Source: CAD feature listing. Evaluate the final solid. Frame: model axes, mm. Face numbers are marked on the shaded views. A direction names the side the tool comes from. Give positions to 0.01 mm unless a question says otherwise; leave off trailing zeros. Loops run counter-clockwise (first coordinate to the right, second up) from the corner with the lowest first, then second, coordinate; pieces in that order, holes last. Notation, with made-up numbers: (56.25, -37.5) - (85.25, -37.5) arc R31 ccw to (85.25, -11.5) - close; hole circle Ø8 at (31.5, -4). An arc over 180 degrees is marked (long way). Put each result on its own line as item: value.
```python
from build123d import *

# Parameters (mm, degrees)
ESBO_O3_W                  = 13.686755529
ESBO_O3_H                  = 42.535935493
ESBO_O4_W                  = 38.680905152
ESBO_O4_H                  = 38.535935493
CORTE_EXTRUS_O1_DEPTH      = 1635.545265364
CORTE_EXTRUS_O1_DEPTH_BACK = 1635.545265364
ESBO_O6_R                  = 34.061990031
ESBO_O7_W                  = 13.69
ESBO_O7_H                  = 42.54
ESBO_O8_W                  = 38.68
ESBO_O8_H                  = 38.54


with BuildPart() as part:
    # Esboço1 → Revolução6 (revolve)
    with BuildSketch(Plane.XY, mode=Mode.PRIVATE) as revolu_o6_sk:
        Polygon((0, 1633), (-35.838224288, 1633), (-35.838224288, 1534.993249603), (-50.245519822, 1534.993249603), (-50.245519822, 1398.116209781), (-35.838224288, 1398.116209781), (-35.838224288, 234.69), (-50.245519822, 234.69), (-50.245519822, 98.01), (-35.838224288, 98.01), (-35.838224288, 0), (0, 0), align=None)
    revolve(revolu_o6_sk.sketch.rotate(Axis((0, 0, 0), (0, 1, 0)), 270), axis=Axis((0, 0, 0), (0, 1, 0)))

    # Esboço3 → Corte-Revolução2 (revolve, cut)
    with BuildSketch(Plane(origin=(0, 0, 0), x_dir=(0, 0, -1), z_dir=(1, 0, 0))):
        with Locations((43.402142058, 1466.554177528)):
            Rectangle(ESBO_O3_W, ESBO_O3_H)
    revolve(axis=Axis((0, 1534.993249603, 0), (0, -1, 0)), mode=Mode.SUBTRACT)

    # Esboço4 → Revolução7 (revolve)
    with BuildSketch(Plane(origin=(0, 0, 0), x_dir=(0, 0, -1), z_dir=(1, 0, 0)), mode=Mode.PRIVATE) as revolu_o7_sk:
        with Locations((19.340452576, 1466.554177528)):
            Rectangle(ESBO_O4_W, ESBO_O4_H)
    revolve(revolu_o7_sk.sketch.rotate(Axis((0, 1487.822145274, 0), (0, -1, 0)), 180), axis=Axis((0, 1487.822145274, 0), (0, -1, 0)))

    # Esboço6 → Corte-extrusão1 (cut, two sides: drawn at the far end of the back side and taken through both)
    with BuildSketch(Plane(origin=(0, 1633, 0), x_dir=(1, 0, 0), z_dir=(0, 1, 0)).offset(-CORTE_EXTRUS_O1_DEPTH_BACK)):
        with Locations(Location((0, 0, 0), (0, 0, 270))):
            Circle(ESBO_O6_R)
    extrude(amount=CORTE_EXTRUS_O1_DEPTH + CORTE_EXTRUS_O1_DEPTH_BACK, mode=Mode.SUBTRACT)

    # Esboço7 → Corte-Revolução3 (revolve, cut)
    with BuildSketch(Plane(origin=(0, 0, 0), x_dir=(0, 0, -1), z_dir=(1, 0, 0)), mode=Mode.PRIVATE) as corte_revolu_o3_sk:
        with Locations((43.400519822, 166.45)):
            Rectangle(ESBO_O7_W, ESBO_O7_H)
    revolve(corte_revolu_o3_sk.sketch.rotate(Axis((0, 234.69, 0), (0, -1, 0)), 180), axis=Axis((0, 234.69, 0), (0, -1, 0)), mode=Mode.SUBTRACT)

    # Esboço8 → Revolução8 (revolve)
    with BuildSketch(Plane.XY, mode=Mode.PRIVATE) as revolu_o8_sk:
        with Locations((19.34, 166.45)):
            Rectangle(ESBO_O8_W, ESBO_O8_H)
    revolve(revolu_o8_sk.sketch.rotate(Axis((0, 145.18, 0), (0, 1, 0)), 270), axis=Axis((0, 145.18, 0), (0, 1, 0)))


solid = part.part
```
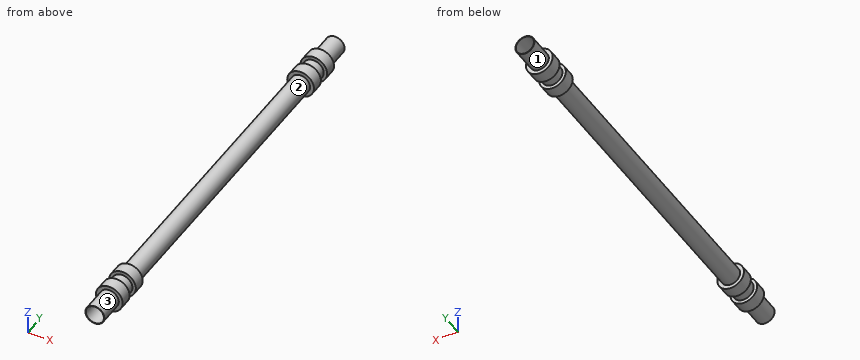
1) Material intervals for line 1 along Y through (x, z) = (46.5, 3); line 2 along Y through (x, z) = (-28, 25); line 3 along X through (y, z) = (1034, 3.5), sorted ascending. Write a range as [from, to].
Check result:
line 1: [98.01, 145.18], [187.72, 234.69], [1398.12, 1445.29], [1487.82, 1534.99]
line 2: [98.01, 145.18], [147.18, 185.72], [187.72, 234.69], [1398.12, 1445.29], [1447.29, 1485.82], [1487.82, 1534.99]
line 3: [-35.67, -33.88], [33.88, 35.67]
2) Pin query (flat end, axial travel): P1, Ø8, axis at x = 15, y = 289.5, coming from the +Z side; P2, Ø23, axis at x = -1, z = -3.5, coming from the -Y side; P3, Ø1.5, axis at x = 24, z = -19, coming from the +Y side; P4, Ø2, axis at y = 496, z = -37, coming from the +X side. Return the tip coordinate at first contact, or that it passes through.
Check result:
P1: z = 34.11
P2: y = 147.18
P3: y = 185.72
P4: through
3) Section query B-B, the plane y = 1517.5. Output: boundary loops of the cut face in (x, z), plus the area to 3 significant figures.
Check result:
outline: circle Ø100.49 at (0, 0); hole circle Ø68.12 at (0, 0)
area: 4,290 mm²
4) Access query for the marked faces 1, 2 and 3. Directions: +Z, -Z, +X, -X, +Y, -Y. A direction counts if a zero-diameter tool reaches every point of the face in a straight line with its end or side. Return the directions, or none.
Check result:
face 1: +Y
face 2: none
face 3: -Y
5) Section query A-A, the plane y = 534.5. Output: boundary loops of the cut face in (x, z), plus the area to 3 significant figures.
Check result:
outline: circle Ø71.68 at (0, 0); hole circle Ø68.12 at (0, 0)
area: 390 mm²
